Could you check a few things on this model? Use its own coordinates, in mm. Face numbers are marked on the shaded views. A direction names the side the tool comes from. Round coordinates to 2 decimals unless told otherwise and drop trailing zeros. Write each loop counter-clockwise with the first axis right and the second up, starting at its lowest first coordinate (ties: lowest second). Pieces come first, ordered by that corner, then holes. Notation, with made-up numbers: (-32, 42) -> (8, 42) arc R18 cw to (8, 72) -> close; hole circle Ø10 at (54.25, 35.5). An arc over 180 degrees is marked (long way). Answer as CSV lines item,"result". Start each with the question number.
Q1. If I drill on line 1 (X direction, y = 5.5, z = 42.5); line 2 (X direction, y = 7.25, z = 36.5); line 3 (Z direction, x = -23, y = 4), over which ranges is the centre line in solid material (lowest first)? Write a range as [from, to].
Q2. Imagine slicing it at A-A on z = 37. Please give me the cut outline in (x, y), and give its area (3 significant figures).
Q3. For the marked faces 1 and 2, which set-ups out of +Z, -Z, +X, -X, +Y, -Y let a thin tool reach every point of the face, with its end or its side?
Q4. Will these pins go through, and if not, where does the flat tip stop? pin 1 Ø2 at (x, z) = (-13.5, 33) entering from -Y; pin 2 Ø10 at (x, y) = (-23, 3.5) entering from +Z.
Q5. Imagine slicing it at C-C on x = -25.4. Please give me the cut outline in (y, z).
Q6. If we mould it in two halves opening along X, with no side actions, what happens to the marked faces 3, 4, 5 and 6? For each: pulls with the +X half, pulls with the -X half, needs draft (parallel to the pull), parting line crosses it, or undercut.
Q7. Imagine slicing it at B-B on x = 25.4. Please give me the cut outline in (y, z), and give its area (3 significant figures).
from build123d import *

# Parameters (mm, degrees)
F0_W     = 101.6
F0_H     = 50.8
F1_DEPTH = 50.8
F2_R     = 12.7
F3_DEPTH = 25.4
F5_R     = 12.7
F4_W     = 101.6
F4_H     = 25.4
F7_DEPTH = 50.8


# Not quite as in the source:
# - an extrude whose draft closes it to a point is written as a loft to that point


with BuildPart() as f1:
    # F0 (on Top) → F1 (new body)
    with BuildSketch(Plane.XY):
        Rectangle(F0_W, F0_H)
    extrude(amount=F1_DEPTH)

    # F2 (on face) → F3 (cut)
    with BuildSketch(Plane.XY.offset(50.8)):
        with Locations((-25.4, 0)):
            Circle(F2_R)
        with Locations((25.4, 0)):
            Circle(F2_R)
    extrude(amount=-F3_DEPTH, mode=Mode.SUBTRACT)

    # F5 (on face) → F6 section 0
    with BuildSketch(Plane.XY.offset(25.4), mode=Mode.PRIVATE) as f6_s0:
        with Locations((25.4, 0)):
            Circle(F5_R)
    loft([f6_s0.sketch, Vertex(25.4, 0, 12.7)], ruled=True, mode=Mode.SUBTRACT)

    # F4 (on face) → F7 (cut, through all)
    with BuildSketch(Plane.XY.offset(50.8)):
        with Locations((0, -12.7)):
            Rectangle(F4_W, F4_H)
    extrude(amount=-F7_DEPTH, mode=Mode.SUBTRACT)


solid = f1.part
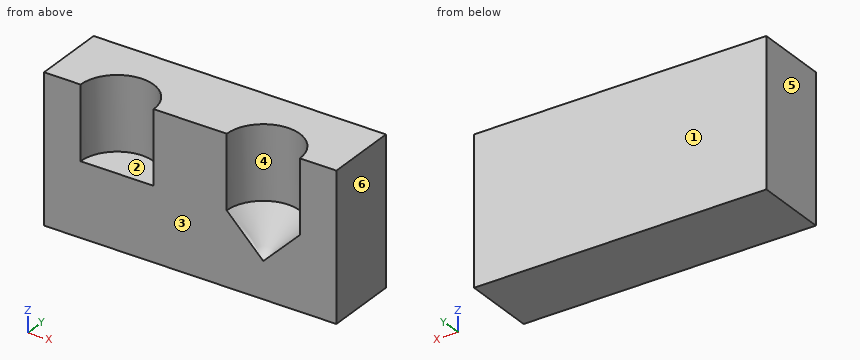
Checks:
1,line 1,"[-50.8, -36.85], [-13.95, 13.95], [36.85, 50.8]"
1,line 2,"[-50.8, -35.83], [-14.97, 14.97], [35.83, 50.8]"
1,line 3,"[0, 25.4]"
2,outline,"(-50.8, 0) -> (-38.1, 0) arc R12.7 cw to (-12.7, 0) -> (12.7, 0) arc R12.7 cw to (38.1, 0) -> (50.8, 0) -> (50.8, 25.4) -> (-50.8, 25.4) -> close"
2,area,"2,070 mm^2"
3,face 1,"+Z, -Z, +X, -X, +Y"
3,face 2,"+Z, -Y"
4,pin 1,"y = 0"
4,pin 2,"z = 25.4"
5,outline,"(0, 0) -> (25.4, 0) -> (25.4, 50.8) -> (12.7, 50.8) -> (12.7, 25.4) -> (0, 25.4) -> close"
6,face 3,"needs draft"
6,face 4,"undercut"
6,face 5,"pulls with the -X half"
6,face 6,"pulls with the +X half"
7,outline,"(0, 0) -> (25.4, 0) -> (25.4, 50.8) -> (12.7, 50.8) -> (12.7, 25.4) -> (0, 12.7) -> close"
7,area,"887 mm^2"
